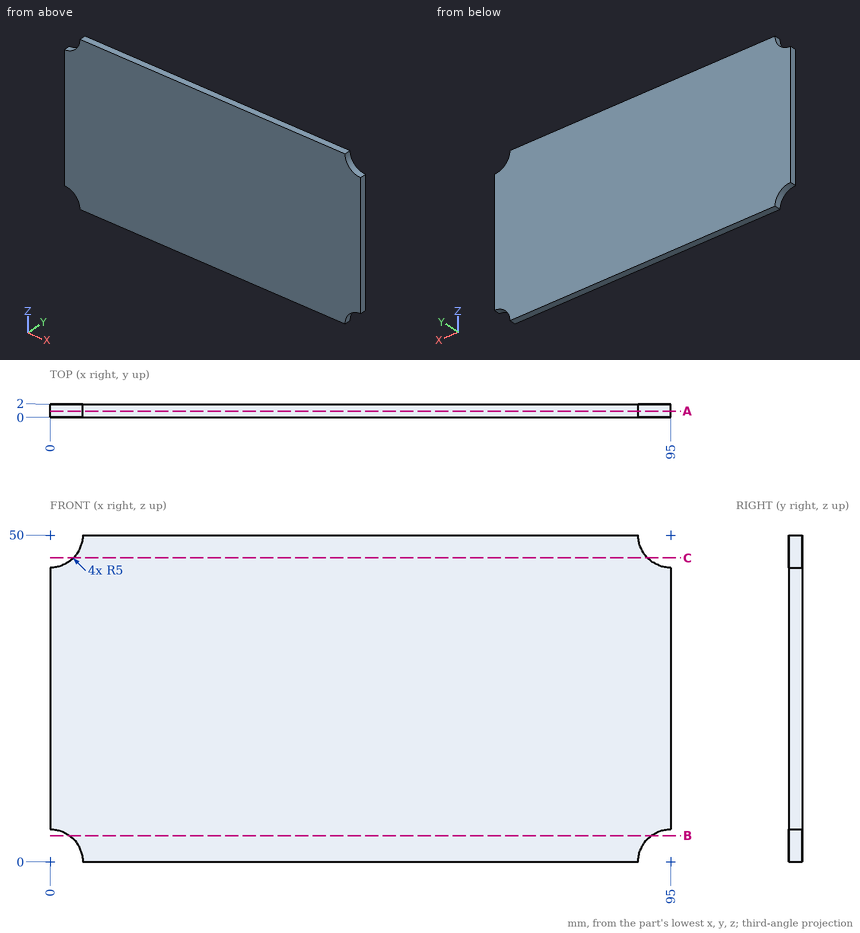
Design review of the part shown in the three views and the two pictorial views. Dimensions are in mm from the part's minimum x, y and z. Coordinates: 2 decimals unless noted, no trailing zeros. Write each loop counter-clockwise with the first axis right and the second up, starting at its lowest first coordinate (ties: lowest second). Pieces come first, ordered by that corner, then holes.
1) We need section A-A on y = 0.9. State the section outline as (x, z) points.
2) We need section C-C on z = 46.5. State the section outline as (x, y) points.
3) To check wall thickness, follow probe 1 along X at (y, z) = (0.3, 47); probe 2 along X at (y, z) = (1.4, 48). State the ranges of each line that lie inside material, in increasing order.
4) We need section B-B on z = 4. State the section outline as (x, y) points, then the cut area to 3 significant figures.
Answer list:
1. outline: (0, 5) arc R5 cw to (5, 0) - (90, 0) arc R5 cw to (95, 5) - (95, 45) arc R5 cw to (90, 50) - (5, 50) arc R5 cw to (0, 45) - close
2. outline: (3.57, 0) - (91.43, 0) - (91.43, 2) - (3.57, 2) - close
3. probe 1: x = 4 to 91
3. probe 2: x = 4.58 to 90.42
4. outline: (3, 0) - (92, 0) - (92, 2) - (3, 2) - close
4. area: 178 mm2
